```python
from build123d import *

# Parameters (mm, degrees)
CYLINDER003006_R     = 1
CYLINDER003006_DEPTH = 20
CYLINDER003003_R     = 2.4
CYLINDER003003_DEPTH = 4.5
CYLINDER003005_R     = 3.45
CYLINDER003005_DEPTH = 4.5


with BuildPart() as cylinder007:
    # Cylinder003006 → Cylinder003006 (new body)
    with BuildSketch(Plane(origin=(11, 10, -8), x_dir=(1, 0, 0), z_dir=(0, 0, 1))):
        Circle(CYLINDER003006_R)
    extrude(amount=CYLINDER003006_DEPTH)


with BuildPart() as cut002002002013:
    # Cylinder003003 → Cylinder003003 (new body)
    with BuildSketch(Plane(origin=(11, 10, -0.5), x_dir=(1, 0, 0), z_dir=(0, 0, 1))):
        Circle(CYLINDER003003_R)
    extrude(amount=CYLINDER003003_DEPTH)

    # Cut002002002013: cut Cylinder007
    add(cylinder007.part, mode=Mode.SUBTRACT)


with BuildPart() as propeller_hub_old:
    # Cylinder003005 → Cylinder003005 (new body)
    with BuildSketch(Plane(origin=(11, 10, -5), x_dir=(1, 0, 0), z_dir=(0, 0, 1))):
        Circle(CYLINDER003005_R)
    extrude(amount=CYLINDER003005_DEPTH)

    # Cut002002002012: cut Cylinder007
    add(cylinder007.part, mode=Mode.SUBTRACT)

    # Connect006: union Cut002002002013
    add(cut002002002013.part)


with BuildPart() as propeller_hub_old_1:
    # Connect006 placement: moved
    add(propeller_hub_old.part.moved(Location((0, 0, 0.5))))


solid = propeller_hub_old_1.part
```
Geometry: final body of the model. Coordinates: model frame, mm. Coordinates: 2 decimals unless noted, no trailing zeros. Order: outer loops, then holes, each group sorted by start corner. A loop starts at its lowest first (then second) coordinate and runs counter-clockwise, first axis right, second up. Notation, with made-up numbers: M -2.75,6.25 L 46.25,6.25 A33 cw 46.25,34.25 Z; hole C 1.5,-35 d9. An arc over 180 degrees is marked long. Answer in a Markdown table with one row per item. Add a question column.
Q1. Contact query for flat-ended pins moving along their axis: P1, Ø1.5, axis at x = 11.5, z = 3.5, coming from the +Y side; P2, Ø1.5, axis at x = 13, z = 2, coming from the +Y side; P3, Ø4, axis at y = 11, z = 2.5, coming from the +X side. Output: stop coordinate, or through.
Q2. Mould query, pull axis X, two halves, no side actions, for faces 1 (the flat face through (13.3, 8.5, 0)), 2 (the cylindrical face through (11, 11, 0)), 3 (the cylindrical face through (10.69, 12.38, 2.22)). Classes: released by +X, released by -X, zero draft, split by the parting line, or undercut.
Q3. Section query B-B on y = 10. Return the cut outline in (x, z), and give its area (4 significant figures).
Q4. Section query C-C on z = -3.25. Return the cut outline in (x, y).
Q5. Section query A-A on x = 11. Return the cut outline in (y, z).
Q6. Line query: L1, parallel to Y at x = 11, z = 0.75; L2, parallel to Y at x = 11, z = -4; L3, parallel to Z at x = 13, y = 11.5. Output: solid intervals per line, ascending.
Q7. Section query D-D on x = 12.5. Return the cut outline in (y, z).
Completed:
| question | item | result |
|---|---|---|
| 1 | P1 | stops at y = 12.4 |
| 1 | P2 | stops at y = 12.05 |
| 1 | P3 | stops at x = 13.4 |
| 2 | face 1 | zero draft |
| 2 | face 2 | undercut |
| 2 | face 3 | split by the parting line |
| 3 | outline | M 7.55,-4.5 L 10,-4.5 L 10,4.5 L 8.6,4.5 L 8.6,0 L 7.55,0 Z; M 12,-4.5 L 14.45,-4.5 L 14.45,0 L 13.4,0 L 13.4,4.5 L 12,4.5 Z |
| 3 | area | 34.65 mm2 |
| 4 | outline | C 11,10 d6.9; hole C 11,10 d2 |
| 5 | outline | M 6.55,-4.5 L 9,-4.5 L 9,4.5 L 7.6,4.5 L 7.6,0 L 6.55,0 Z; M 11,-4.5 L 13.45,-4.5 L 13.45,0 L 12.4,0 L 12.4,4.5 L 11,4.5 Z |
| 6 | L1 | y = 7.6 to 9, 11 to 12.4 |
| 6 | L2 | y = 6.55 to 9, 11 to 13.45 |
| 6 | L3 | z = -4.5 to 0 |
| 7 | outline | M 6.89,-4.5 L 13.11,-4.5 L 13.11,0 L 11.87,0 L 11.87,4.5 L 8.13,4.5 L 8.13,0 L 6.89,0 Z |
